from build123d import *

# Parameters (mm, degrees)
BOSS_EXTRUDE1_DEPTH = 20
CUT_EXTRUDE1_DEPTH  = 5
SKETCH3_R           = 2.25
CUT_EXTRUDE2_DEPTH  = 15


with BuildPart() as part:
    # Sketch1 → Boss-Extrude1 (new body, symmetric)
    with BuildSketch(Plane.XY):
        with BuildLine():
            Line((0, 0), (22.5, 0))
            Line((22.5, 0), (17.5, 5))
            Line((17.5, 5), (72.5, 5))
            Line((72.5, 5), (67.5, 0))
            Line((67.5, 0), (90, 0))
            Line((90, 0), (90, 15))
            Line((90, 15), (80, 15))
            Line((80, 15), (80, 25))
            Line((80, 25), (70, 25))
            ThreePointArc((70, 25), (62.5, 17.5), (55, 25))
            Line((55, 25), (35, 25))
            ThreePointArc((35, 25), (27.5, 17.5), (20, 25))
            Line((20, 25), (10, 25))
            Line((10, 25), (10, 15))
            Line((10, 15), (0, 15))
            Line((0, 15), (0, 0))
        make_face()
    extrude(amount=BOSS_EXTRUDE1_DEPTH, both=True)

    # Sketch2 → Cut-Extrude1 (cut)
    with BuildSketch(Plane.XY.offset(20)):
        with BuildLine():
            Line((17.5, 5), (37.5, 5))
            Line((37.5, 5), (37.5, 12.5))
            Line((37.5, 12.5), (27.5, 12.5))
            ThreePointArc((27.5, 12.5), (18.661165235, 16.161165235), (15, 25))
            Line((15, 25), (10, 25))
            Line((10, 25), (10, 15))
            Line((10, 15), (0, 15))
            Line((0, 15), (0, 0))
            Line((0, 0), (22.5, 0))
            Line((22.5, 0), (17.5, 5))
        make_face()
        with BuildLine():
            Line((62.5, 12.5), (52.5, 12.5))
            Line((52.5, 12.5), (52.5, 5))
            Line((52.5, 5), (72.5, 5))
            Line((72.5, 5), (67.5, 0))
            Line((67.5, 0), (90, 0))
            Line((90, 0), (90, 15))
            Line((90, 15), (80, 15))
            Line((80, 15), (80, 25))
            Line((80, 25), (75, 25))
            ThreePointArc((75, 25), (71.338834765, 16.161165235), (62.5, 12.5))
        make_face()
    cut_extrude1 = extrude(amount=-CUT_EXTRUDE1_DEPTH, mode=Mode.SUBTRACT)

    # Mirror1: Cut-Extrude1 across plane
    add(cut_extrude1.mirror(Plane.XY), mode=Mode.SUBTRACT)

    # Sketch3 → Cut-Extrude2 (cut)
    with BuildSketch(Plane(origin=(0, 25, 0), x_dir=(1, 0, 0), z_dir=(0, 1, 0))):
        with Locations((45, 15)):
            Circle(SKETCH3_R)
        with Locations((45, -15)):
            Circle(SKETCH3_R)
        with Locations((75, 7.5)):
            Circle(SKETCH3_R)
        with Locations((75, -7.5)):
            Circle(SKETCH3_R)
        with Locations((15, 7.5)):
            Circle(SKETCH3_R)
        with Locations((15, -7.5)):
            Circle(SKETCH3_R)
    extrude(amount=-CUT_EXTRUDE2_DEPTH, mode=Mode.SUBTRACT)


solid = part.part
Here's how the part is built. I have some questions about the finished solid (model axes, mm). A direction names the side the tool comes from. Coordinates: 2 decimals unless noted, no trailing zeros. Order: outer loops, then holes, each group sorted by start corner. A loop starts at its lowest first (then second) coordinate and runs counter-clockwise, first axis right, second up. Notation, with made-up numbers: (-29.5, -16) -> (-11.5, -16) arc R17 ccw to (-11.5, 0) -> close; hole circle Ø11 at (36.5, -26). An arc over 180 degrees is marked (long way). Answer in a Markdown table with one row per item.
(1) Will these pins go through, and if not, where does the flat tip stop? pin 1 Ø2 at (x, z) = (74.5, -6.5) entering from +Y; pin 2 Ø3 at (y, z) = (22, -1.5) entering from -X; pin 3 Ø5.5 at (x, z) = (30.5, -18) entering from -Y.
Answer key:
| item | result |
|---|---|
| pin 1 | y = 10 |
| pin 2 | x = 10 |
| pin 3 | y = 12.5 |
(2) I want a section at B-B on y = 23.25. Count the separate pieces of the cut face and the enclosed holes in it, then the cut area to 3 significant figures.
Answer key:
| item | result |
|---|---|
| separate pieces | 3 |
| enclosed holes | 6 |
| area | 1,440 mm^2 |
(3) I want a section at A-A on x = 54. List the corners of the cut face in (y, z) for me, then the cut area to 3 significant figures.
Answer key:
| item | result |
|---|---|
| outline | (5, -15) -> (12.5, -15) -> (12.5, -20) -> (25, -20) -> (25, 20) -> (12.5, 20) -> (12.5, 15) -> (5, 15) -> close |
| area | 725 mm^2 |
(4) I want a section at D-D on y = 14. List the corners of the cut face in (x, z) for me.
Answer key:
| item | result |
|---|---|
| outline | (0, -15) -> (21.56, -15) -> (21.56, -20) -> (68.44, -20) -> (68.44, -15) -> (90, -15) -> (90, 15) -> (68.44, 15) -> (68.44, 20) -> (21.56, 20) -> (21.56, 15) -> (0, 15) -> close; hole circle Ø4.5 at (15, -7.5); hole circle Ø4.5 at (15, 7.5); hole circle Ø4.5 at (45, -15); hole circle Ø4.5 at (45, 15); hole circle Ø4.5 at (75, -7.5); hole circle Ø4.5 at (75, 7.5) |
(5) I want a section at C-C on z = 7.5. List the corners of the cut face in (x, y) for me.
Answer key:
| item | result |
|---|---|
| outline | (0, 0) -> (22.5, 0) -> (17.5, 5) -> (72.5, 5) -> (67.5, 0) -> (90, 0) -> (90, 15) -> (80, 15) -> (80, 25) -> (77.25, 25) -> (77.25, 10) -> (72.75, 10) -> (72.75, 25) -> (70, 25) arc R7.5 cw to (55, 25) -> (35, 25) arc R7.5 cw to (20, 25) -> (17.25, 25) -> (17.25, 10) -> (12.75, 10) -> (12.75, 25) -> (10, 25) -> (10, 15) -> (0, 15) -> close |
(6) Please list where these lines run through material, in increasing order: probe 1 along X at (y, z) = (17, -7.5); probe 2 along Z at (x, y) = (75, 20.5); probe 3 along Z at (x, y) = (45, 16.5).
Answer key:
| item | result |
|---|---|
| probe 1 | 10 to 12.75, 17.25 to 72.75, 77.25 to 80 |
| probe 2 | -15 to -9.75, -5.25 to 5.25, 9.75 to 15 |
| probe 3 | -20 to -17.25, -12.75 to 12.75, 17.25 to 20 |
(7) On a 3-axis mill with a long thin cutter (end or side, diameter ignored), from which of +Z, -Z, +X, -X, +Y, -Y can I reach the whole of each face in a straight line? I mean faces 1 (the face through (5, 15, 0)), 2 (the face through (18.759, 16.065, 17.535)), 3 (the face through (15, 10, 7)). Say none if no direction works.
Answer key:
| item | result |
|---|---|
| face 1 | +Z, -Z, -X, +Y |
| face 2 | +Z, -X, -Y |
| face 3 | +Y |
(8) Thinking about a two-plate mould opening in X: for faces 4 (the face through (52.5, 9, -18)), 5 (the face through (45, 10, -15)), 6 (the face through (11, 0, 0)), which applies, +X half, -X half, draft (parallel to the pull), parting line (faces both ways), or undercut?
Answer key:
| item | result |
|---|---|
| face 4 | +X half |
| face 5 | undercut |
| face 6 | draft |
